The figure shows three views and two pictorial views of one solid part (mm, origin at its lowest corner). Answer the questions. A direction names the side the tool comes from. Coordinates: 2 decimals unless noted, no trailing zeros. Loops run counter-clockwise (first coordinate to the right, second up) from the corner with the lowest first, then second, coordinate; pieces in that order, holes last. Notation, with made-up numbers: (43, 41.5) -> (50, 41.5) arc R22 ccw to (50, 49.5) -> close; hole circle Ø1 at (47, 44). An arc over 180 degrees is marked (long way). Answer as a JSON object with one key per item and string values. Group by question number.
1) Section B-B, the plane z = 300 is taken. Give the vertices of the cut face in (x, y).
2) Section C-C, the plane y = 300 is taken. Give the vertices of the cut face in (x, z), plus the area to 3 significant figures.
3) Consider probe 1 along Y at (x, z) = (228, 300); probe 2 along Y at (x, z) = (109.5, 318.5); probe 3 along X at (y, z) = (110, 364). Determine where each line is inside the solid, lowest interval first. Write a range as [from, to].
4) Flat-ended cylindrical pins translate along their axes: P1, Ø5, axis at x = 184.5, y = 119.5, coming from the -Z side; P2, Ø4, axis at x = 129, y = 81.5, coming from the -Z side; P3, Ø4, axis at x = 225.5, y = 420, coming from the +Z side. Find the tip coordinate at first contact, or state that the pin passes through.
5) Section A-A, the plane x = 241 is taken. Give the vertices of the cut face in (y, z), plus the area to 3 significant figures.
6) Section D-D, the plane x = 158 is taken. Give the vertices of the cut face in (y, z).
7) Determine the mould class of the marked faces 1, 2, 3 and 4 for opening direction Y: released by +Y, released by -Y, zero draft, split by the parting line, or undercut.
8) Which of the six approach directions +Z, -Z, +X, -X, +Y, -Y give full straight-line access (tool end or side, diameter ignored) to the marked faces 5, 6 and 7?
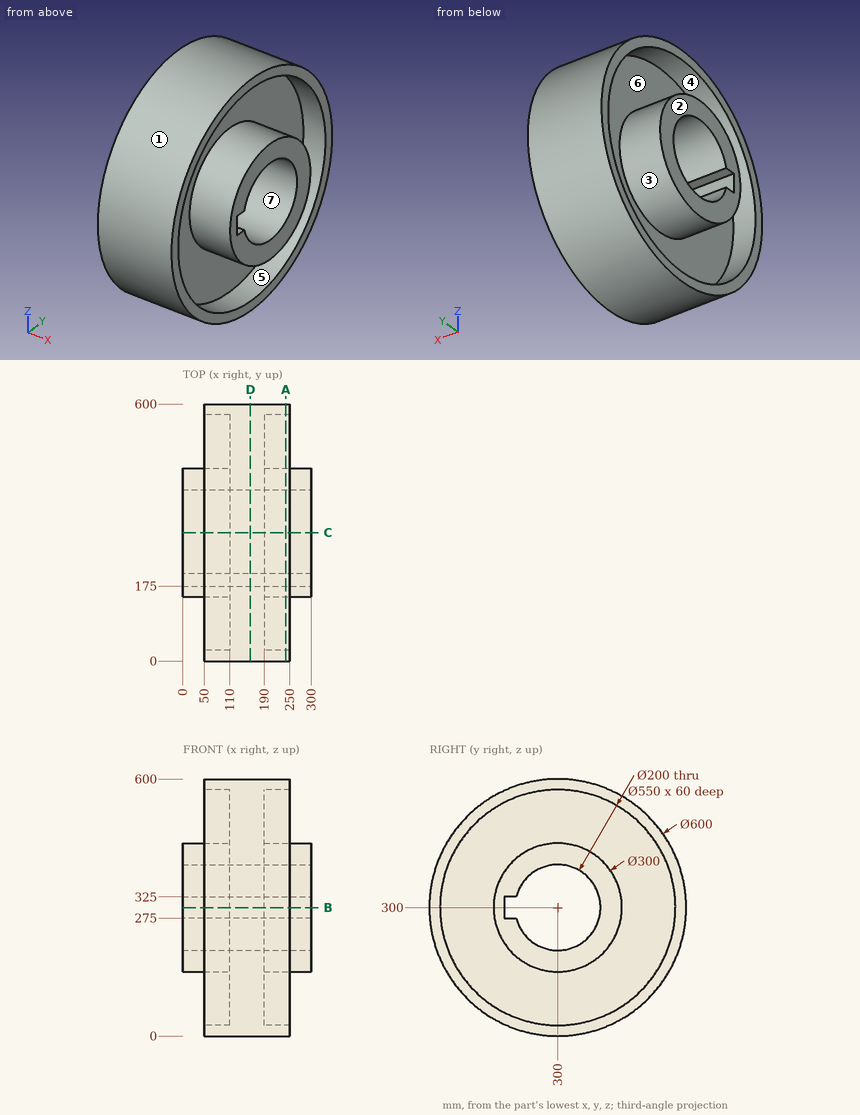
Determined:
{
 "1": {"outline": "(0, 150) -> (110, 150) -> (110, 25) -> (50, 25) -> (50, 0) -> (250, 0) -> (250, 25) -> (190, 25) -> (190, 150) -> (300, 150) -> (300, 175) -> (0, 175) -> close; (0, 400) -> (300, 400) -> (300, 450) -> (190, 450) -> (190, 575) -> (250, 575) -> (250, 600) -> (50, 600) -> (50, 575) -> (110, 575) -> (110, 450) -> (0, 450) -> close"},
 "2": {"outline": "(0, 150) -> (110, 150) -> (110, 25) -> (50, 25) -> (50, 0) -> (250, 0) -> (250, 25) -> (190, 25) -> (190, 150) -> (300, 150) -> (300, 200) -> (0, 200) -> close; (0, 400) -> (300, 400) -> (300, 450) -> (190, 450) -> (190, 575) -> (250, 575) -> (250, 600) -> (50, 600) -> (50, 575) -> (110, 575) -> (110, 450) -> (0, 450) -> close", "area": "60,000 mm²"},
 "3": {"probe 1": "[0, 25], [150, 175], [400, 450], [575, 600]", "probe 2": "[0.57, 25.62], [151.15, 175], [398.27, 448.85], [574.38, 599.43]", "probe 3": "[110, 190]"},
 "4": {"P1": "z = 58.51", "P2": "z = 92.33", "P3": "z = 575.82"},
 "5": {"outline": "circle Ø600 at (300, 300); circle Ø300 at (300, 300); hole circle Ø550 at (300, 300); hole (175, 275) -> (203.18, 275) arc R100 ccw (long way) to (203.18, 325) -> (175, 325) -> close", "area": "83,100 mm²"},
 "6": {"outline": "circle Ø600 at (300, 300); hole (175, 275) -> (203.18, 275) arc R100 ccw (long way) to (203.18, 325) -> (175, 325) -> close"},
 "7": {"face 1": "split by the parting line", "face 2": "zero draft", "face 3": "undercut", "face 4": "undercut"},
 "8": {"face 5": "+X", "face 6": "-X", "face 7": "+X, -X"}
}
